Geometry: final body of the model. Coordinates: model frame, mm. A direction names the side the tool comes from. Give positions to 0.01 mm unless a question says otherwise; leave off trailing zeros. Write each loop counter-clockwise with the first axis right and the second up, starting at its lowest first coordinate (ties: lowest second). Pieces come first, ordered by that corner, then holes.
from build123d import *

# Parameters (mm, degrees)
F0_R     = 25
F0_R_2   = 4
F1_DEPTH = 2.5


with BuildPart() as f1:
    # F0 (on Front) → F1 (new body, symmetric)
    with BuildSketch(Plane.XZ):
        Circle(F0_R)
        with BuildLine():
            Line((-11.274977, -12.283114), (-3.309475, -7.684229))
            ThreePointArc((-3.309475, -7.684229), (-2.912357, -7.555561), (-2.497311, -7.600226))
            ThreePointArc((-2.497311, -7.600226), (0, -8), (2.497311, -7.600226))
            ThreePointArc((2.497311, -7.600226), (2.912357, -7.555561), (3.309475, -7.684229))
            Line((3.309475, -7.684229), (11.274977, -12.283114))
            ThreePointArc((11.274977, -12.283114), (11.771663, -13.067786), (11.4088, -13.922618))
            ThreePointArc((11.4088, -13.922618), (0, -18), (-11.4088, -13.922618))
            ThreePointArc((-11.4088, -13.922618), (-11.771663, -13.067786), (-11.274977, -12.283114))
        make_face(mode=Mode.SUBTRACT)
        with BuildLine():
            ThreePointArc((-17.761741, -2.919001), (-15.588457, 9), (-6.352941, 16.841619))
            ThreePointArc((-6.352941, 16.841619), (-5.431203, 16.728452), (-5, 15.905974))
            Line((-5, 15.905974), (-5, 6.708204))
            ThreePointArc((-5, 6.708204), (-5.087129, 6.299956), (-5.333333, 5.962848))
            ThreePointArc((-5.333333, 5.962848), (-6.928203, 4), (-7.830644, 1.637378))
            ThreePointArc((-7.830644, 1.637378), (-7.999486, 1.255605), (-8.309475, 0.976025))
            Line((-8.309475, 0.976025), (-16.274977, -3.62286))
            ThreePointArc((-16.274977, -3.62286), (-17.202866, -3.660666), (-17.761741, -2.919001))
        make_face(mode=Mode.SUBTRACT)
        Circle(F0_R_2, mode=Mode.SUBTRACT)
        with BuildLine():
            ThreePointArc((5.333333, 5.962848), (5.087129, 6.299956), (5, 6.708204))
            Line((5, 6.708204), (5, 15.905974))
            ThreePointArc((5, 15.905974), (5.431204, 16.728452), (6.352941, 16.841619))
            ThreePointArc((6.352941, 16.841619), (15.588457, 9), (17.761741, -2.919001))
            ThreePointArc((17.761741, -2.919001), (17.202866, -3.660666), (16.274977, -3.62286))
            Line((16.274977, -3.62286), (8.309475, 0.976025))
            ThreePointArc((8.309475, 0.976025), (7.999486, 1.255605), (7.830644, 1.637378))
            ThreePointArc((7.830644, 1.637378), (6.928203, 4), (5.333333, 5.962848))
        make_face(mode=Mode.SUBTRACT)
    extrude(amount=F1_DEPTH, both=True)

    # F2 (on Right) → F3 (revolve, cut)
    with BuildSketch(Plane.YZ):
        Polygon((-2, 25), (0, 21), (0, 25), align=None)
        Polygon((0, 25), (0, 21), (2, 25), align=None)
    revolve(axis=Axis((0, 0.001726, 0), (0, 1, 0)), mode=Mode.SUBTRACT)


solid = f1.part
Q1. Pull-direction query (Z, two-part tool) for faces 4 (the cylindrical face through (23.09, 2.25, -9.58)), 5 (the flat face through (5, 2.5, 0)), 6 (the cylindrical face through (-5.442, -0.035, 16.736)); classes: released by +Z, released by -Z, zero draft, split by the parting line, or undercut.
Filled sheet:
face 4: split by the parting line
face 5: zero draft
face 6: undercut
Q2. Ray query, line 1 along Z through (x, y) = (-6, 2.05); line 2 along X through (y, z) = (-2.15, -1); line 3 along Z through (x, y) = (-3.5, 0.65). Return the intervals inside material, ascending.
Filled sheet:
line 1: z = -24.27 to -16.97, -9.24 to 5.29, 16.91 to 24.27
line 2: x = -24.98 to -17.97, -11.73 to -3.87, 3.87 to 11.73, 17.97 to 24.98
line 3: z = -22.02 to -17.66, -7.79 to -1.94, 1.94 to 22.02
Q3. Section A-A on z = 0. Output: boundary loops of the cut face in (x, y), plus the area to 3 significant figures.
Filled sheet:
outline: (-25, -2.5) - (-18, -2.5) - (-18, 2.5) - (-25, 2.5) - (-25, 2) - (-21, 0) - (-25, -2) - close; (-10, -2.5) - (-4, -2.5) - (-4, 2.5) - (-10, 2.5) - close; (4, -2.5) - (10, -2.5) - (10, 2.5) - (4, 2.5) - close; (18, -2.5) - (25, -2.5) - (25, -2) - (21, 0) - (25, 2) - (25, 2.5) - (18, 2.5) - close
area: 114 mm2
Q4. Pin query (flat end, axial travel): P1, Ø3, axis at y = -1, z = -3, coming from the -X side; P2, Ø13, axis at x = 0, z = 0, coming from the -Y side; P3, Ø3, axis at x = 7, z = -12.5, coming from the -Y side; P4, Ø1.5, axis at y = -1, z = 10, coming from the +X side. Return the tip coordinate at first contact, or that it passes through.
Filled sheet:
P1: stops at x = -24.93
P2: stops at y = -2.5
P3: passes through
P4: stops at x = 22.4
Q5. Section C-C on z = 14.5. Count the separate pieces of the cut face and the enclosed holes in it, plus the area to 3 significant figures.
Filled sheet:
separate pieces: 3
enclosed holes: 0
area: 127 mm2
Q6. Section B-B on x = 0. Output: boundary loops of the cut face in (y, z), plus the area to 3 significant figures.
Filled sheet:
outline: (-2.5, -25) - (-2, -25) - (0, -21) - (2, -25) - (2.5, -25) - (2.5, -18) - (-2.5, -18) - close; (-2.5, -8) - (2.5, -8) - (2.5, -4) - (-2.5, -4) - close; (-2.5, 4) - (2.5, 4) - (2.5, 25) - (2, 25) - (0, 21) - (-2, 25) - (-2.5, 25) - close
area: 144 mm2
Q7. Access query for faces 1 (the flat face through (5, -2.5, 0)), 2 (the conical face through (6.383, 0.125, 20.269)), 3 (the cylindrical face through (-17.191, -0.035, -3.666)). Directions: +Z, -Z, +X, -X, +Y, -Y. A direction counts if a zero-diameter tool reaches every point of the face in a straight line with its end or side. Return the directions, or none.
Filled sheet:
face 1: +Z, -Z, +X, -X, -Y
face 2: none
face 3: +Y, -Y
